For this review, use the dimensioned drawing (mm, ordinates from the lowest corner) and the shaded views. A direction names the side the tool comes from. Round coordinates to 2 decimals unless told otherwise and drop trailing zeros. Write each loop counter-clockwise with the first axis right and the second up, starting at its lowest first coordinate (ties: lowest second). Pieces come first, ordered by that corner, then holes. Notation, with made-up numbers: M 22,43 L 59,43 A23 cw 59,69 Z; hole C 87.25,-16 d11. An arc over 180 degrees is marked long. One line per question, with ' | ' between items.
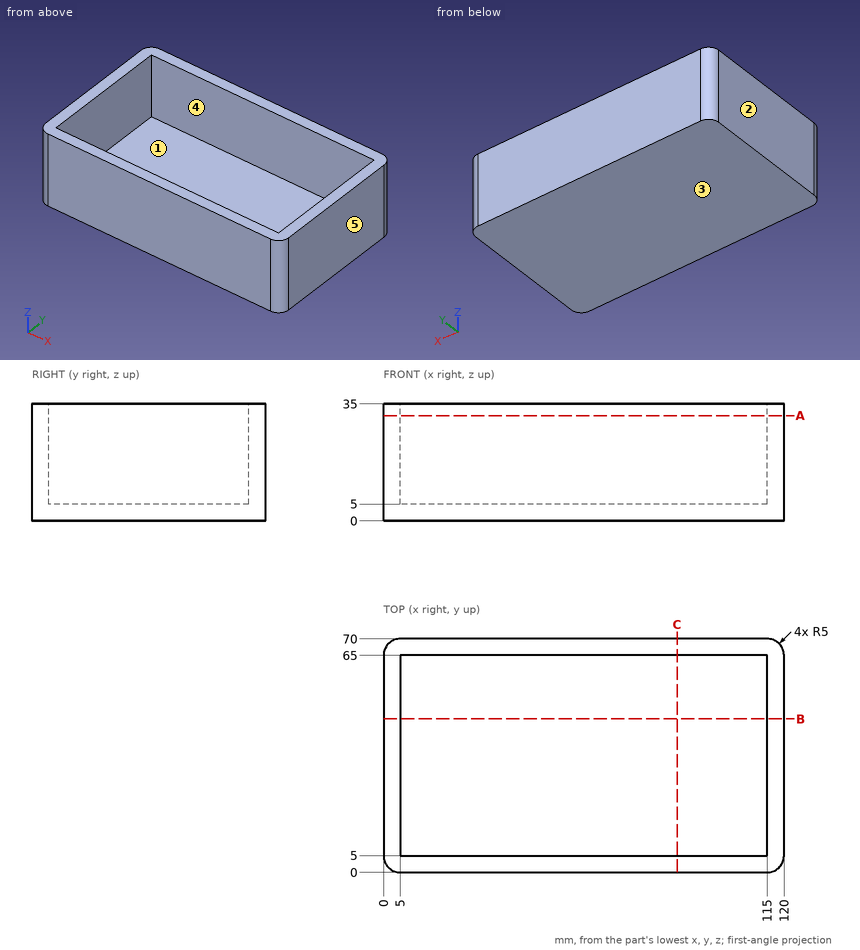
Item 1: Mouldability with a two-part tool opening along X and no side actions: class the marked faces 3, 4 and 5 as +X half, -X half, draft (parallel to the pull), parting line (faces both ways), or undercut.
Results:
face 3: draft | face 4: undercut | face 5: +X half
Item 2: Insertion check: pin 1 Ø15 at (y, z) = (39, 21) entering from -X; pin 2 Ø2 at (x, y) = (91.5, 21) entering from +Z. Each pin has a flat end and moves straight along its axis. Give the tip position at first contact, or say it passes through.
Results:
pin 1: x = 0 | pin 2: z = 5
Item 3: Take a section at C-C (x = 88). Write out the cut boundary in (y, z), then the cut area to 3 significant figures.
Results:
outline: M 0,0 L 70,0 L 70,35 L 65,35 L 65,5 L 5,5 L 5,35 L 0,35 Z | area: 650 mm2
Item 4: To check wall thickness, follow line 1 along X through (y, z) = (29, 25.5); line 2 along Y through (x, z) = (6, 22.5); line 3 along Z through (x, y) = (75, 44.5). State the ranges of each line that lie inside material, in increasing order. Write a range as from..to.
Results:
line 1: 0..5, 115..120 | line 2: 0..5, 65..70 | line 3: 0..5
Item 5: Take a section at B-B (y = 46). Write out the cut boundary in (x, z).
Results:
outline: M 0,0 L 120,0 L 120,35 L 115,35 L 115,5 L 5,5 L 5,35 L 0,35 Z
Item 6: Take a section at A-A (z = 31.5). Write out the cut boundary in (x, y).
Results:
outline: M 0,5 A5 ccw 5,0 L 115,0 A5 ccw 120,5 L 120,65 A5 ccw 115,70 L 5,70 A5 ccw 0,65 Z; hole M 5,5 L 115,5 L 115,65 L 5,65 Z
Item 7: Machinability: for the marked faces 1 and 2, which of the approach directions +Z, -Z, +X, -X, +Y, -Y give a long, thin tool a straight path to every point of the face, cutting with its end or side? Answer none if there is none.
Results:
face 1: +Z | face 2: +Z, -Z, -X, +Y, -Y
